```python
from build123d import *

# Parameters (mm, degrees)
CROQUIS2_R              = 20
SALIENTE_EXTRUIR1_DEPTH = 80
CORTAR_EXTRUIR1_REACH   = 82
CROQUIS3_W              = 10
CROQUIS3_H              = 80
CROQUIS3_W_2            = 20
CROQUIS4_R              = 25
SALIENTE_EXTRUIR2_DEPTH = 30
CROQUIS5_R              = 25
SALIENTE_EXTRUIR3_DEPTH = 30


with BuildPart() as part:
    # Croquis2 → Saliente-Extruir1 (new body)
    with BuildSketch(Plane(origin=(0, 0, 0), x_dir=(0, 0, -1), z_dir=(1, 0, 0))):
        with BuildLine():
            Line((0, 0), (80, 0))
            Line((80, 0), (80, 120))
            ThreePointArc((80, 120), (40, 160), (0, 120))
            Line((0, 120), (0, 0))
        make_face()
        with Locations((40, 120)):
            Circle(CROQUIS2_R, mode=Mode.SUBTRACT)
    extrude(amount=-SALIENTE_EXTRUIR1_DEPTH)

    # Croquis3 → Cortar-Extruir1 (cut, up to next)
    with BuildSketch(Plane.XY, mode=Mode.PRIVATE) as cortar_extruir1_sk1:
        with Locations((-5, 120)):
            Rectangle(CROQUIS3_W, CROQUIS3_H)
    cortar_extruir1_tool1 = extrude(cortar_extruir1_sk1.sketch, amount=-CORTAR_EXTRUIR1_REACH, mode=Mode.PRIVATE) & part.part
    add(cortar_extruir1_tool1.solids().sort_by_distance((-5, 120, 0))[0], mode=Mode.SUBTRACT)
    # Croquis3 → Cortar-Extruir1 (cut, up to next)
    with BuildSketch(Plane.XY, mode=Mode.PRIVATE) as cortar_extruir1_sk2:
        with Locations((-75, 120)):
            Rectangle(CROQUIS3_W, CROQUIS3_H)
    cortar_extruir1_tool2 = extrude(cortar_extruir1_sk2.sketch, amount=-CORTAR_EXTRUIR1_REACH, mode=Mode.PRIVATE) & part.part
    add(cortar_extruir1_tool2.solids().sort_by_distance((-75, 120, 0))[0], mode=Mode.SUBTRACT)
    # Croquis3 → Cortar-Extruir1 (cut, up to next)
    with BuildSketch(Plane.XY, mode=Mode.PRIVATE) as cortar_extruir1_sk3:
        with Locations((-40, 120)):
            Rectangle(CROQUIS3_W_2, CROQUIS3_H)
    cortar_extruir1_tool3 = extrude(cortar_extruir1_sk3.sketch, amount=-CORTAR_EXTRUIR1_REACH, mode=Mode.PRIVATE) & part.part
    add(cortar_extruir1_tool3.solids().sort_by_distance((-40, 120, 0))[0], mode=Mode.SUBTRACT)

    # Croquis4 → Saliente-Extruir2 (add)
    with BuildSketch(Plane.XY):
        with Locations((-40, 35)):
            Circle(CROQUIS4_R)
    extrude(amount=SALIENTE_EXTRUIR2_DEPTH)

    # Croquis5 → Saliente-Extruir3 (add)
    with BuildSketch(Plane(origin=(0, 0, -80), x_dir=(-1, 0, 0), z_dir=(0, 0, -1))):
        with Locations((40, 35)):
            Circle(CROQUIS5_R)
    extrude(amount=SALIENTE_EXTRUIR3_DEPTH)


solid = part.part
```
The listing builds one solid part. Answer for the finished solid, in the listing's coordinates (mm). A direction names the side the tool comes from. Round coordinates to 2 decimals unless told otherwise and drop trailing zeros. Loops run counter-clockwise (first coordinate to the right, second up) from the corner with the lowest first, then second, coordinate; pieces in that order, holes last. Notation, with made-up numbers: (70.5, 26.5) - (79.5, 26.5) arc R31 cw to (79.5, 61.5) - close; hole circle Ø4 at (30.5, -13). An arc over 180 degrees is marked (long way). Return JSON: item names as keys, results as strings. Group by question number.
1. Consider probe 1 along X at (y, z) = (91, -2.5); probe 2 along Y at (x, z) = (-20, -40); probe 3 along Z at (x, y) = (-46.5, 72). Determine where each line is inside the solid, lowest interval first.
2. Each of these flat-tipped pins is pushed along its axis until it touches: P1, Ø6, axis at x = -31.5, y = 129, coming from the -Z side; P2, Ø24, axis at y = 127, z = -57, coming from the +X side; P3, Ø10, axis at x = -30.5, z = -75, coming from the +Y side. Where does it stop, or does it pass through?
3. The part is cut by section D-D on x = -40. Determine the outline of the cut face in (y, z).
4. The mould has two halves that part along X. Classify faces 1 (the flat face through (-40, 35, 30)), 2 (the flat face through (-50, 101.7, -30.6)), 3 (the flat face through (0, 41, -39)), 4 (the flat face through (-40, 80, -39)): pulls with the +X half, pulls with the -X half, needs draft (parallel to the pull), parting line crosses it, or undercut.
5. The part is cut by section A-A on x = -55. Determine the outline of the cut face in (y, z), then the cut area to 3 significant figures.
6. The part is cut by section B-B on z = -40. Determine the outline of the cut face in (x, y).
7. The part is cut by section C-C on y = 35. Determine the outline of the cut face in (x, z).
8. Which of the six approach directions +Z, -Z, +X, -X, +Y, -Y give full straight-line access (tool end or side, diameter ignored) to faces 5 (the cylindrical face through (-60, 20, 15)), 6 (the flat face through (-75, 80, -39)), 7 (the flat face through (-10, 101.7, -30.6)), 8 (the cylindrical face through (-63.09, 25.42, -94.79))?
Resolved:
{
 "1": {"probe 1": "x = -70 to -50, -30 to -10", "probe 2": "y = 0 to 100, 140 to 160", "probe 3": "z = -80 to 0"},
 "2": {"P1": "stops at z = -79.48", "P2": "stops at x = -10", "P3": "stops at y = 146.43"},
 "3": {"outline": "(0, -80) - (10, -80) - (10, -110) - (60, -110) - (60, -80) - (80, -80) - (80, 0) - (60, 0) - (60, 30) - (10, 30) - (10, 0) - (0, 0) - close"},
 "4": {"face 1": "needs draft", "face 2": "undercut", "face 3": "pulls with the +X half", "face 4": "undercut"},
 "5": {"outline": "(0, -80) - (15, -80) - (15, -110) - (55, -110) - (55, -80) - (120, -80) arc R40 ccw to (120, 0) - (55, 0) - (55, 30) - (15, 30) - (15, 0) - (0, 0) - close; hole circle Ø40 at (120, -40)", "area": "13,300 mm²"},
 "6": {"outline": "(-80, 0) - (0, 0) - (0, 80) - (-10, 80) - (-10, 100) - (-30, 100) - (-30, 80) - (-50, 80) - (-50, 100) - (-70, 100) - (-70, 80) - (-80, 80) - close; (-70, 140) - (-50, 140) - (-50, 160) - (-70, 160) - close; (-30, 140) - (-10, 140) - (-10, 160) - (-30, 160) - close"},
 "7": {"outline": "(-80, -80) - (-65, -80) - (-65, -110) - (-15, -110) - (-15, -80) - (0, -80) - (0, 0) - (-15, 0) - (-15, 30) - (-65, 30) - (-65, 0) - (-80, 0) - close"},
 "8": {"face 5": "+Z", "face 6": "+Z, -Z, -X, +Y", "face 7": "+Z, -Z, +X, +Y", "face 8": "-Z"}
}
